Design review of the part built by this model. Coordinates are the model's own, in mm. A direction names the side the tool comes from. Give positions to 0.01 mm unless a question says otherwise; leave off trailing zeros. Loops run counter-clockwise (first coordinate to the right, second up) from the corner with the lowest first, then second, coordinate; pieces in that order, holes last. Notation, with made-up numbers: M 85.5,3 L 115.5,3 A22 cw 115.5,18 Z; hole C -32,84.5 d3. An arc over 180 degrees is marked long. Use a Markdown table: item, result. Add a question column.
(1) Add section C-C, the plane z = 0. Give the boundary of the cut face in (x, y), then the cut area to 3 significant figures.
(2) Draft analysis for pull direction X (two halves, no side actions). For faces 3 (the face through (11, 2.96, 11.07)), 4 (the face through (-11, 2.96, -11.07)), 5 (the face through (-9.644, 2.958, 6.825)), state which applies: pulls with the +X half, pulls with the -X half, needs draft (parallel to the pull), parting line crosses it, or undercut.
(3) Insertion check: pin 1 Ø3.5 at (x, z) = (0, 0) entering from +Y. The pin has a flat end and moves straight along its axis. Give the tip position at first contact, or say it passes through.
(4) For faces 1 (the face through (0, 3, 12.5)), 2 (the face through (0, 3, -0.8)), list the 3-axis set-ups (+Z, -Z, +X, -X, +Y, -Y) from which the entire face can be reached by the end or side of a thin tool; tool diameter is ignored.
(5) For probe 1 along Z at (x, y) = (7.5, 4.25); probe 2 along Z at (x, y) = (-9.5, 0.35); probe 3 along Z at (x, y) = (0, 1.5), list the stretches that pass through material, from the lowest coordinate up.
(6) Add section D-D, the plane z = 5.75. Give the boundary of the cut face in (x, y), then the cut area to 3 significant figures.
(7) Add section A-A, the plane x = 0. Give the boundary of the cut face in (y, z), then the cut area to 3 significant figures.
(8) Add section B-B, the plane y = 1.2. Give the boundary of the cut face in (x, z), then the cut area to 3 significant figures.
```python
from build123d import *

# Parameters (mm, degrees)
BOSS_EXTRUDE1_DEPTH   = 6
F_8_CLEARANCE_HOLE1_D = 4.4958


with BuildPart() as part:
    # Sketch1 → Boss-Extrude1 (new body)
    with BuildSketch(Plane(origin=(0, 0, 0), x_dir=(1, 0, 0), z_dir=(0, 1, 0))):
        with BuildLine():
            Line((7.5, 12.5), (-7.5, 12.5))
            ThreePointArc((-7.5, 12.5), (-11.035533906, 11.035533906), (-12.5, 7.5))
            Line((-12.5, 7.5), (-12.5, -7.5))
            ThreePointArc((-12.5, -7.5), (-11.035533906, -11.035533906), (-7.5, -12.5))
            Line((-7.5, -12.5), (7.5, -12.5))
            ThreePointArc((7.5, -12.5), (11.035533906, -11.035533906), (12.5, -7.5))
            Line((12.5, -7.5), (12.5, 7.5))
            ThreePointArc((12.5, 7.5), (11.035533906, 11.035533906), (7.5, 12.5))
        make_face()
        with BuildLine():
            Line((-1.833030278, 0.8), (1.833030278, 0.8))
            ThreePointArc((1.833030278, 0.8), (0, -2), (-1.833030278, 0.8))
        make_face(mode=Mode.SUBTRACT)
    extrude(amount=BOSS_EXTRUDE1_DEPTH)

    # #8 Clearance Hole1 (through all)
    with Locations(Plane(origin=(0, 6, 0), x_dir=(1, 0, 0), z_dir=(0, 1, 0))):
        with Locations((-7.5, 7.5), (7.5, 7.5), (-7.5, -7.5), (7.5, -7.5)):
            Hole(F_8_CLEARANCE_HOLE1_D / 2)


solid = part.part
```
Established:
| question | item | result |
|---|---|---|
| 1 | outline | M -12.5,0 L -2,0 L -2,6 L -12.5,6 Z; M 2,0 L 12.5,0 L 12.5,6 L 2,6 Z |
| 1 | area | 126 mm^2 |
| 2 | face 3 | pulls with the +X half |
| 2 | face 4 | pulls with the -X half |
| 2 | face 5 | undercut |
| 3 | pin 1 | y = 6 |
| 4 | face 1 | +Z, +X, -X, +Y, -Y |
| 4 | face 2 | +Y, -Y |
| 5 | probe 1 | -12.5 to -9.75, -5.25 to 5.25, 9.75 to 12.5 |
| 5 | probe 2 | -12.08 to -8.53, -6.47 to 6.47, 8.53 to 12.08 |
| 5 | probe 3 | -12.5 to -0.8, 2 to 12.5 |
| 6 | outline | M -12.5,0 L -8.91,0 L -8.91,6 L -12.5,6 Z; M -6.09,0 L 6.09,0 L 6.09,6 L -6.09,6 Z; M 8.91,0 L 12.5,0 L 12.5,6 L 8.91,6 Z |
| 6 | area | 116 mm^2 |
| 7 | outline | M 0,-12.5 L 6,-12.5 L 6,-0.8 L 0,-0.8 Z; M 0,2 L 6,2 L 6,12.5 L 0,12.5 Z |
| 7 | area | 133 mm^2 |
| 8 | outline | M -12.5,-7.5 A5 ccw -7.5,-12.5 L 7.5,-12.5 A5 ccw 12.5,-7.5 L 12.5,7.5 A5 ccw 7.5,12.5 L -7.5,12.5 A5 ccw -12.5,7.5 Z; hole C -7.5,-7.5 d4.5; hole C -7.5,7.5 d4.5; hole M -1.83,-0.8 L 1.83,-0.8 A2 ccw long Z; hole C 7.5,-7.5 d4.5; hole C 7.5,7.5 d4.5 |
| 8 | area | 531 mm^2 |
